Design review of the part built by this model. Coordinates are the model's own, in mm. A direction names the side the tool comes from. Round coordinates to 2 decimals unless told otherwise and drop trailing zeros. Order: outer loops, then holes, each group sorted by start corner. A loop starts at its lowest first (then second) coordinate and runs counter-clockwise, first axis right, second up. Notation, with made-up numbers: M 8.5,-6 L 24.5,-6 A12 ccw 24.5,2 Z; hole C -23,67 d8. An arc over 180 degrees is marked long. Use a Markdown table: item, result. Add a question column.
(1) The part is to be moulded in two halves that separate along Z. For faces 1 (the face through (10, 12.5, 2)), 2 (the face through (0, 11, 0)), 3 (the face through (5.859, 11.03, 3.077)), say which applies: released by +Z, released by -Z, zero draft, split by the parting line, or undercut.
(2) Machinability: for faces 4 (the face through (-7.26, 12.35, 0.7)), 5 (the face through (9.75, 0, 3)), which of the approach directions +Z, -Z, +X, -X, +Y, -Y give a long, thin tool a straight path to every point of the face, cutting with its end or side? Answer none if there is none.
(3) Take a section at B-B (x = 4.75). Write out the cut boundary in (y, z), then the cut area to 4 significant figures.
(4) Take a section at D-D (x = 0.75). Write out the cut boundary in (y, z), then the cut area to 3 significant figures.
(5) Take a section at A-A (z = 0.5). Count the separate pieces of the cut face and the enclosed holes in it, then the cut area to 3 significant figures.
(6) For pin 1 (3 mm diameter, centred on x = 11.5, y = -1.5, fed in from -Z); pin 2 (1.7 mm diameter, centred on x = -12.25, y = 10.25, fed in from -Z); pin 3 (2.5 mm diameter, centred on y = -3, z = 2, fed in from -X), all flat-tipped, find the tip position at first contact; note any pin that passes through.
(7) To check wall thickness, follow probe 1 along Z at (x, y) = (-7.25, 10); probe 2 along X at (y, z) = (-11.4, 2.5); probe 3 along X at (y, z) = (11.6, 2.5). State the ranges of each line that lie inside material, in increasing order. Write a range as from..to.
(8) Take a section at C-C (y = -10.25). Write out the cut boundary in (x, z).
Autodesk Inventor part; units mm, degrees
ref_plane "YZ Plane" through (0, 0, 0) normal (1, 0, 0) x (0, 1, 0)
ref_plane "XZ Plane" through (0, 0, 0) normal (0, 1, 0) x (-1, 0, 0)
ref_plane "XY Plane" through (0, 0, 0) normal (0, 0, 1) x (1, 0, 0)
sketch "スケッチ1" plane through (0, 0, 0) normal (0, 0, 1) x (1, 0, 0)
  line L0 (-14.75, -12.5) -> (14.75, -12.5)
  line L1 (14.75, -12.5) -> (14.75, 12.5)
  line L2 (14.75, 12.5) -> (-14.75, 12.5)
  line L3 (-14.75, 12.5) -> (-14.75, -12.5)
  line L4 (-14.75, -12.5) -> (14.75, 12.5) construction
  line L5 (14.75, -12.5) -> (-14.75, 12.5) construction
  point P0 (0, 0)
  dimension "d0" = 29.5
  dimension "d1" = 25
extrude "プレート1" add sketch "スケッチ1" along normal blind 5
sketch "スケッチ2" plane through (0, 0, 5) normal (0, 0, 1) x (1, 0, 0)
  line L0 (-12.25, -10.25) -> (12.75, -10.25) construction
  line L1 (12.75, -10.25) -> (12.75, 10.25) construction
  line L2 (12.75, 10.25) -> (-12.25, 10.25) construction
  line L3 (-12.25, 10.25) -> (-12.25, -10.25) construction
  line L4 (-12.25, -10.25) -> (12.75, 10.25) construction
  line L5 (12.75, -10.25) -> (-12.25, 10.25) construction
  line L6 (14.75, 12.5) -> (14.75, -12.5) construction
  point P0 (0, 0)
  point P1 (0.25, 0)
  dimension "d3" = 25
  dimension "d4" = 20.5
  dimension "d5" = 2
hole "穴1" at (-12.25, 10.25, 5) at (12.75, 10.25, 5) at (12.75, -10.25, 5) at (-12.25, -10.25, 5) direction (0, 0, -1) diameter 2.1 end through all
sketch "スケッチ3" plane through (0, 0, 0) normal (0, 0, -1) x (-1, 0, 0)
  line L0 (-14.75, -12.5) -> (-14.75, 12.5)
  line L1 (14.75, 12.5) -> (14.75, -12.5)
  line L2 (-14.75, 7.7) -> (14.75, 7.7)
  line L3 (14.75, -7.7) -> (-14.75, -7.7)
  line L4 (-14.75, 12.5) -> (14.75, 12.5)
  line L5 (14.75, -12.5) -> (-14.75, -12.5)
  point P0 (0, 0)
  dimension "d13" = 4.8
  dimension "d14" = 4.8
extrude "押し出し1" cut sketch "スケッチ3" against normal blind 1.5 contours L0 L2 L1 L3
sketch "スケッチ4" plane through (0, 0, 5) normal (0, 0, 1) x (1, 0, 0)
  line L0 (-14.75, 12.5) -> (14.75, 12.5)
  line L1 (14.75, -12.5) -> (-14.75, -12.5)
  circle A0 centre (-20.25, 0) radius 11.5
  line L2 (14.75, 12.5) -> (14.75, -12.5)
  line L3 (9.75, -9.6) -> (-9.25, -9.6)
  line L4 (-9.25, -9.6) -> (-9.25, 9.6)
  line L5 (-9.25, 9.6) -> (9.75, 9.6)
  line L6 (9.75, 9.6) -> (9.75, -9.6)
  line L7 (9.75, -9.6) -> (-9.25, 9.6) construction
  line L8 (-9.25, -9.6) -> (9.75, 9.6) construction
  line L9 (-9.25, 7.7) -> (-11.7083, 7.7)
  line L10 (-11.7083, 7.7) -> (-11.7083, -7.7)
  line L11 (-11.7083, -7.7) -> (-9.25, -7.7)
  line L12 (-9.25, -7.7) -> (-9.25, 7.7)
  line L13 (14.75, 7.7) -> (-14.75, 7.7)
  point P0 (0, 0)
  point P1 (14.75, 0)
  point P2 (0.25, 0)
  point P3 (-9.25, 0)
  point P4 (-11.7083, 7.7)
  dimension "d18" = 23
  dimension "d17" = 35
  dimension "d19" = 5
  dimension "d20" = 2.9
  dimension "d22" = 19
extrude "押し出し2" cut sketch "スケッチ4" against normal through all
fillet "フィレット1" radius 1 14 edges at (-9.25, 9.6, 2.5) (-9.25, -9.6, 2.5) (9.75, -9.6, 2.5) (9.75, 9.6, 2.5) (-9.25, 7.7, 2.5) (-9.25, -7.7, 2.5) (-11.7083, -7.7, 2.5) (-11.7083, 7.7, 2.5) (-14.75, -10.0995, 2.5) (-14.75, 10.0995, 2.5) (-14.75, -12.5, 2.5) (14.75, -12.5, 2.5) (14.75, 12.5, 2.5) (-14.75, 12.5, 2.5)
sketch "スケッチ5" plane through (0, 0, 5) normal (0, 0, 1) x (1, 0, 0)
  line L0 (-13.75, 12.5) -> (13.75, 12.5)
  circle A0 centre (-7.25, 13.4) radius 1.05
  circle A1 centre (4.75, 13.4) radius 1.05
  line L1 (14.75, 11.5) -> (14.75, -11.5)
  point P0 (0, 0)
  dimension "d26" = 2.1
  dimension "d27" = 2.1
  dimension "d28" = 0.9
  dimension "d29" = 0.9
  dimension "d30" = 12
  dimension "d31" = 10
extrude "押し出し3" cut sketch "スケッチ5" against normal through all
sketch "スケッチ6" plane through (-6.7092, 12.5, 0) normal (0, 1, 0) x (1, 0, 0)
  line L0 (-1.0817, -5) -> (-1.0817, 0)
  line L1 (0, -5) -> (-1.0817, -5)
  line L2 (0, 0) -> (0, -5)
  line L3 (-1.0817, 0) -> (0, 0)
  line L4 (10.9183, -5) -> (10.9183, 0)
  line L5 (12, -5) -> (10.9183, -5)
  line L6 (12, 0) -> (12, -5)
  line L7 (10.9183, 0) -> (12, 0)
  line L8 (-1.5408, -5) -> (-1.5408, 0) construction
  line L9 (-1.5408, 0) -> (-1.5408, -5) construction
  line L10 (-1.0817, -2.5) -> (0, -2.5) construction
  line L11 (10.9183, -2.5) -> (12, -2.5) construction
  line L12 (11.4592, -5) -> (11.4592, 0) construction
  point P0 (6.7092, 0)
  point P1 (-0.5408, -2.5)
  point P2 (11.4592, -2.5)
hole "穴2" at (-7.25, 12.5, 2.5) at (4.75, 12.5, 2.5) direction (0, -1, 0) diameter 2.5 end through all
mirror "ミラー1" about plane through (0, 0, 0) normal (0, 1, 0) of "穴2", "押し出し3"
equation "\"d11\" = Thickness"
equation "\"d14\" = d13"
equation "\"d29\" = d28"
equation "\"d2\" = Thickness"
equation "\"BendRadius\" = Thickness"
equation "\"BendReliefWidth\" = Thickness"
equation "\"BendReliefDepth\" = 0.5 * Thickness"
equation "\"TransitionRadius\" = BendRadius"
equation "\"JacobiRadiusSize\" = BendRadius"
equation "\"GapSize\" = Thickness"
properties part number "T3.0_servo-mount_3D プリント"
Verdict:
| question | item | result |
|---|---|---|
| 1 | face 1 | zero draft |
| 1 | face 2 | released by -Z |
| 1 | face 3 | undercut |
| 2 | face 4 | +Z, -Z, +Y |
| 2 | face 5 | +Z, -Z |
| 3 | outline | M -12.35,0 L -9.6,0 L -9.6,1.25 L -12.35,1.25 Z; M -12.35,3.75 L -9.6,3.75 L -9.6,5 L -12.35,5 Z; M 9.6,0 L 12.35,0 L 12.35,1.25 L 9.6,1.25 Z; M 9.6,3.75 L 12.35,3.75 L 12.35,5 L 9.6,5 Z |
| 3 | area | 13.75 mm^2 |
| 4 | outline | M -12.5,0 L -9.6,0 L -9.6,5 L -12.5,5 Z; M 9.6,0 L 12.5,0 L 12.5,5 L 9.6,5 Z |
| 4 | area | 29.0 mm^2 |
| 5 | separate pieces | 2 |
| 5 | enclosed holes | 4 |
| 5 | area | 188 mm^2 |
| 6 | pin 1 | stops at z = 1.5 |
| 6 | pin 2 | passes through |
| 6 | pin 3 | stops at x = 9.75 |
| 7 | probe 1 | z = 0..1.25, 3.75..5 |
| 7 | probe 2 | x = -14.75..-8.5, -6..3.5, 6..14.75 |
| 7 | probe 3 | x = -14.74..-8.5, -6..3.5, 6..14.74 |
| 8 | outline | M -14.65,0 L -13.3,0 L -13.3,5 L -14.65,5 Z; M -11.2,0 L 11.7,0 L 11.7,5 L -11.2,5 Z; M 13.8,0 L 14.75,0 L 14.75,5 L 13.8,5 Z; hole C -7.25,2.5 d2.5; hole C 4.75,2.5 d2.5 |
